```python
from build123d import *

# Parameters (mm, degrees)
SKETCH1_W           = 152.4
SKETCH1_H           = 101.6
BOSS_EXTRUDE1_DEPTH = 12.7
SKETCH2_R           = 5
CUT_EXTRUDE1_DEPTH  = 12.7
SKETCH3_R           = 3.175
CUT_EXTRUDE2_DEPTH  = 93.457395594


with BuildPart() as part:
    # Sketch1 → Boss-Extrude1 (new body)
    with BuildSketch(Plane(origin=(0, 0, 0), x_dir=(1, 0, 0), z_dir=(0, 1, 0))):
        Rectangle(SKETCH1_W, SKETCH1_H)
    extrude(amount=BOSS_EXTRUDE1_DEPTH)

    # Sketch2 → Cut-Extrude1 (cut)
    with BuildSketch(Plane.XZ):
        with Locations(Location((-50.004206057, 21.825, 0), (0, 0, 270))):
            Circle(SKETCH2_R)
        with Locations(Location((-50.004206057, -21.825, 0), (0, 0, 270))):
            Circle(SKETCH2_R)
        with Locations(Location((-0.004206057, 21.825, 0), (0, 0, 270))):
            Circle(SKETCH2_R)
        with Locations(Location((-0.004206057, -21.825, 0), (0, 0, 270))):
            Circle(SKETCH2_R)
        with Locations(Location((49.995793943, 21.825, 0), (0, 0, 270))):
            Circle(SKETCH2_R)
        with Locations(Location((49.995793943, -21.825, 0), (0, 0, 270))):
            Circle(SKETCH2_R)
    extrude(amount=-CUT_EXTRUDE1_DEPTH, mode=Mode.SUBTRACT)

    # Sketch3 → Cut-Extrude2 (cut, through all)
    with BuildSketch(Plane(origin=(0, 12.7, 0), x_dir=(1, 0, 0), z_dir=(0, 1, 0))):
        with Locations(Location((-63.5, -38.1, 0), (0, 0, 270))):
            Circle(SKETCH3_R)
        with Locations(Location((-38.1, -38.1, 0), (0, 0, 270))):
            Circle(SKETCH3_R)
        with Locations(Location((-12.7, -38.1, 0), (0, 0, 270))):
            Circle(SKETCH3_R)
        with Locations(Location((12.7, -38.1, 0), (0, 0, 270))):
            Circle(SKETCH3_R)
        with Locations(Location((38.1, -38.1, 0), (0, 0, 270))):
            Circle(SKETCH3_R)
        with Locations(Location((63.5, -38.1, 0), (0, 0, 270))):
            Circle(SKETCH3_R)
        with Locations(Location((-38.1, 38.1, 0), (0, 0, 270))):
            Circle(SKETCH3_R)
        with Locations(Location((-12.7, 38.1, 0), (0, 0, 270))):
            Circle(SKETCH3_R)
        with Locations(Location((12.7, 38.1, 0), (0, 0, 270))):
            Circle(SKETCH3_R)
        with Locations(Location((38.1, 38.1, 0), (0, 0, 270))):
            Circle(SKETCH3_R)
        with Locations(Location((63.5, 38.1, 0), (0, 0, 270))):
            Circle(SKETCH3_R)
        with Locations(Location((-63.5, 38.1, 0), (0, 0, 270))):
            Circle(SKETCH3_R)
    extrude(amount=-CUT_EXTRUDE2_DEPTH, mode=Mode.SUBTRACT)


solid = part.part
```
Geometry check sheet. Reference: the model listing, model coordinates, mm. Round coordinates to 2 decimals unless told otherwise and drop trailing zeros. Order: outer loops, then holes, each group sorted by start corner. A loop starts at its lowest first (then second) coordinate and runs counter-clockwise, first axis right, second up. Notation, with made-up numbers: (59.5, 46.25) - (105.5, 46.25) arc R28 cw to (105.5, 81.25) - close; hole circle Ø11 at (-21.5, 59). An arc over 180 degrees is marked (long way). Use a Markdown table: item, result. Add a question column.
(1) Material ranges on line 1 along Z through (x, y) = (-13, 12); line 2 along Z through (x, y) = (-50, 4.75) (3 decimals), recorded low to high. Write a range as [from, to].
(2) Sectioned sample at A-A, the plane z = 38.1. Enter the section's corners in (x, y) (3 decimals).
(3) Depth check by flat-ended pin: pin 1 (4 mm diameter, centred on x = -63.5, z = 38.1, fed in from +Y). Enter the tip coordinate at first touch or a pass-through.
(4) Release check for a two-part mould opening along X. For faces 1 (the cylindrical face through (-63.36, 6.44, -41.27)), 2 (the flat face through (-76.2, 6, 1)), 3 (the flat face through (-1, 12.7, -1)), 4 (the cylindrical face through (1.498, 6.261, 17.056)) record: pulls with the +X half, pulls with the -X half, needs draft (parallel to the pull), parting line crosses it, or undercut.
(5) Sectioned sample at C-C, the plane y = 3. Count the separate pieces of the cut face and the enclosed holes in it, and give its area (3 significant figures).
(6) Sectioned sample at B-B, the plane x = 63.5. Enter the section's corners in (y, z) (3 decimals).
Answers below:
| question | item | result |
|---|---|---|
| 1 | line 1 | [-50.8, -41.26], [-34.94, 34.94], [41.26, 50.8] |
| 1 | line 2 | [-50.8, -26.825], [-16.825, 16.825], [26.825, 50.8] |
| 2 | outline | (-76.2, 0) - (-66.675, 0) - (-66.675, 12.7) - (-76.2, 12.7) - close; (-60.325, 0) - (-41.275, 0) - (-41.275, 12.7) - (-60.325, 12.7) - close; (-34.925, 0) - (-15.875, 0) - (-15.875, 12.7) - (-34.925, 12.7) - close; (-9.525, 0) - (9.525, 0) - (9.525, 12.7) - (-9.525, 12.7) - close; (15.875, 0) - (34.925, 0) - (34.925, 12.7) - (15.875, 12.7) - close; (41.275, 0) - (60.325, 0) - (60.325, 12.7) - (41.275, 12.7) - close; (66.675, 0) - (76.2, 0) - (76.2, 12.7) - (66.675, 12.7) - close |
| 3 | pin 1 | through |
| 4 | face 1 | undercut |
| 4 | face 2 | pulls with the -X half |
| 4 | face 3 | needs draft |
| 4 | face 4 | undercut |
| 5 | separate pieces | 1 |
| 5 | enclosed holes | 18 |
| 5 | area | 14,600 mm² |
| 6 | outline | (0, -50.8) - (12.7, -50.8) - (12.7, -41.275) - (0, -41.275) - close; (0, -34.925) - (12.7, -34.925) - (12.7, 34.925) - (0, 34.925) - close; (0, 41.275) - (12.7, 41.275) - (12.7, 50.8) - (0, 50.8) - close |
